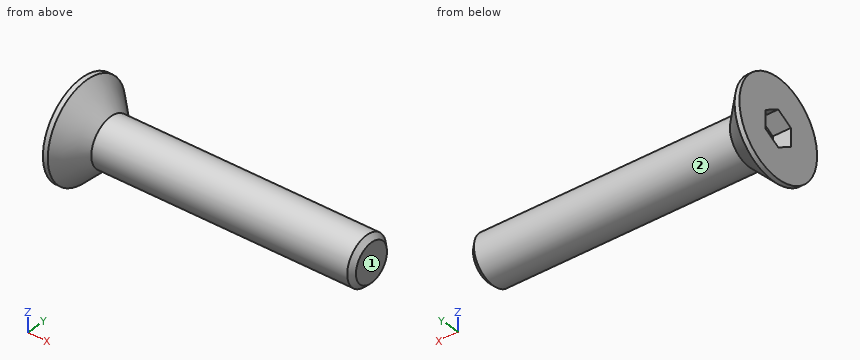
from build123d import *

# Parameters (mm, degrees)
CHAMFER1_SIZE      = 0.2
CUT_EXTRUDE1_DEPTH = 0.75


with BuildPart() as part:
    # Sketch1 → Revolve1 (revolve)
    with BuildSketch(Plane.XY):
        Polygon((0, 1), (-1, 2), (-1.2, 2), (-1.2, 0), (10.8, 0), (10.8, 1), align=None)
    revolve(axis=Axis((-1.2, 0, 0), (1, 0, 0)))

    # Chamfer1
    chamfer1_edges = [part.edges().sort_by_distance(p)[0] for p in [
        (10.8, -1, 0),
    ]]
    chamfer(chamfer1_edges, length=CHAMFER1_SIZE)

    # Sketch2 → Cut-Extrude1 (cut)
    with BuildSketch(Plane.ZY.offset(1.2)):
        Polygon((-0.75055535, 0), (-0.375277675, -0.65), (0.375277675, -0.65), (0.75055535, 0), (0.375277675, 0.65), (-0.375277675, 0.65), align=None)
    extrude(amount=-CUT_EXTRUDE1_DEPTH, mode=Mode.SUBTRACT)


solid = part.part
Work out the finished part from the listing and answer in its coordinate system (mm). Face numbers are marked on the shaded views. A direction names the side the tool comes from. Round coordinates to 2 decimals unless told otherwise and drop trailing zeros. Write each loop counter-clockwise with the first axis right and the second up, starting at its lowest first coordinate (ties: lowest second). Pieces come first, ordered by that corner, then holes.
1) A cutting plane is placed at A-A (z = 0). Give the vertices of the cut face in (x, y), plus the area to 3 significant figures.
2) A cutting plane is placed at B-B (x = 9.25). Give the vertices of the cut face in (y, z).
3) A tool of negligible diameter and unlimited length cuts with its end or side. For the marked faces 1 and 2, from which of +Z, -Z, +X, -X, +Y, -Y can it reach the whole face along a straight path? Write none if from no direction.
4) Straight lines are drawn through the part: line 1 (X direction, y = 0.4, z = 0.2); line 2 (Y direction, x = -0.25, z = 0.1); line 3 (Z direction, x = 8.5, y = -0.7). For each, find the intervals that lie inside material, in ascending order.
5) Given pin 1 Ø1 at (x, z) = (9, 0) entering from -Y, flat-ended and moving along its own axis, determine where the tip first touches the part or whether it passes through.
Completed:
1. outline: (-1.2, -2) - (-1, -2) - (0, -1) - (10.6, -1) - (10.8, -0.8) - (10.8, 0.8) - (10.6, 1) - (0, 1) - (-1, 2) - (-1.2, 2) - (-1.2, 0.65) - (-0.45, 0.65) - (-0.45, -0.65) - (-1.2, -0.65) - close
1. area: 24.4 mm2
2. outline: circle Ø2 at (0, 0)
3. face 1: +Z, -Z, +X, +Y, -Y
3. face 2: +X
4. line 1: x = -0.45 to 10.8
4. line 2: y = -1.25 to 1.25
4. line 3: z = -0.71 to 0.71
5. pin 1: stops at y = -1
